from build123d import *

# Parameters (mm, degrees)
SKETCH1_R                    = 8
BOSS_EXTRUDE1_DEPTH          = 0.5
SKETCH2_R                    = 6.1
CUT_EXTRUDE1_DEPTH           = 1.5
F_1_0_1_DIAMETER_HOLE1_D     = 1
F_1_0_1_DIAMETER_HOLE1_DEPTH = 0.5


with BuildPart() as part:
    # Sketch1 → Boss-Extrude1 (new body)
    with BuildSketch(Plane(origin=(0, 0, 0), x_dir=(1, 0, 0), z_dir=(0, 1, 0))):
        Circle(SKETCH1_R)
    extrude(amount=BOSS_EXTRUDE1_DEPTH)

    # Sketch2 → Cut-Extrude1 (cut, through all)
    with BuildSketch(Plane(origin=(0, 0.5, 0), x_dir=(1, 0, 0), z_dir=(0, 1, 0))):
        Circle(SKETCH2_R)
    extrude(amount=-CUT_EXTRUDE1_DEPTH, mode=Mode.SUBTRACT)

    # Ø1.0 (1) Diameter Hole1
    with Locations(Plane(origin=(0, 0.5, 0), x_dir=(1, 0, 0), z_dir=(0, 1, 0))):
        with Locations((-7, 0), (7, 0)):
            Hole(F_1_0_1_DIAMETER_HOLE1_D / 2, depth=F_1_0_1_DIAMETER_HOLE1_DEPTH)


solid = part.part
For this review, take the finished solid that the model builds, in its own axes (mm). Coordinates: 2 decimals unless noted, no trailing zeros. Write each loop counter-clockwise with the first axis right and the second up, starting at its lowest first coordinate (ties: lowest second). Pieces come first, ordered by that corner, then holes. Notation, with made-up numbers: (22, 23.5) -> (44, 23.5) arc R21 ccw to (44, 62.5) -> close; hole circle Ø9 at (71.5, 65). An arc over 180 degrees is marked (long way). Write each question's results on one line, items separated by ' | '. Start each with the question number.
1) Consider section A-A (z = 0). Write out the cut boundary in (x, y), plus the area to 3 significant figures.
2) Wall thickness on L1, parallel to Z at x = 0, y = 0.45; L2, parallel to Z at x = -2.5, y = 0.4; L3, parallel to X at y = 0.15, z = -1.75: over which ranges is each line inside the solid? List them lowest first. Write a range as [from, to].
3) Consider section D-D (z = 5.5). Write out the cut boundary in (x, y), plus the area to 3 significant figures.
4) Consider section B-B (x = -7). Write out the cut boundary in (y, z).
5) Consider section C-C (y = 0.3). Write out the cut boundary in (x, z), plus the area to 3 significant figures.
6) The part is to be moulded in two halves that separate along Z. For faces 1 (the face through (2, 0, 6)), 2 (the face through (-7.477, 0.246, -0.15)), 3 (the face through (-1.73, 0.25, 7.81)), say which applies: +Z half, -Z half, draft (parallel to the pull), parting line (faces both ways), or undercut.
Geometry says:
1) outline: (-8, 0) -> (-7.5, 0) -> (-7.5, 0.5) -> (-8, 0.5) -> close; (-6.5, 0) -> (-6.1, 0) -> (-6.1, 0.5) -> (-6.5, 0.5) -> close; (6.1, 0) -> (6.5, 0) -> (6.5, 0.5) -> (6.1, 0.5) -> close; (7.5, 0) -> (8, 0) -> (8, 0.5) -> (7.5, 0.5) -> close | area: 0.900 mm^2
2) L1: [-8, -6.1], [6.1, 8] | L2: [-7.6, -5.56], [5.56, 7.6] | L3: [-7.81, -5.84], [5.84, 7.81]
3) outline: (-5.81, 0) -> (-2.64, 0) -> (-2.64, 0.5) -> (-5.81, 0.5) -> close; (2.64, 0) -> (5.81, 0) -> (5.81, 0.5) -> (2.64, 0.5) -> close | area: 3.17 mm^2
4) outline: (0, -3.87) -> (0.5, -3.87) -> (0.5, -0.5) -> (0, -0.5) -> close; (0, 0.5) -> (0.5, 0.5) -> (0.5, 3.87) -> (0, 3.87) -> close
5) outline: circle Ø16 at (0, 0); hole circle Ø1 at (-7, 0); hole circle Ø12.2 at (0, 0); hole circle Ø1 at (7, 0) | area: 82.6 mm^2
6) face 1: draft | face 2: undercut | face 3: parting line
